```python
from build123d import *

# Parameters (mm, degrees)
SALIENTE_EXTRUIR1_DEPTH = 60
CORTAR_EXTRUIR1_REACH   = 50
CROQUIS2_R              = 2
CROQUIS2_R_2            = 12.5
SALIENTE_EXTRUIR2_DEPTH = 15
CROQUIS4_W              = 60
CROQUIS4_H              = 6
SALIENTE_EXTRUIR3_DEPTH = 1
CORTAR_EXTRUIR2_REACH   = 50
CROQUIS5_R              = 2.75
CROQUIS6_R              = 6
CORTAR_EXTRUIR3_DEPTH   = 8
REDONDEO1_R             = 5


with BuildPart() as part:
    # Croquis1 → Saliente-Extruir1 (new body)
    with BuildSketch(Plane.XY):
        Polygon((0, 0), (0, -30), (42, -30), (42, -90), (48, -90), (48, -21), (14, -21), (14, 0), align=None)
    extrude(amount=SALIENTE_EXTRUIR1_DEPTH)

    # Croquis2 → Cortar-Extruir1 (cut, up to next)
    with BuildSketch(Plane(origin=(48, 0, 0), x_dir=(0, 0, -1), z_dir=(1, 0, 0)), mode=Mode.PRIVATE) as cortar_extruir1_sk1:
        with Locations((-45.5, -44.5)):
            Circle(CROQUIS2_R)
    cortar_extruir1_tool1 = extrude(cortar_extruir1_sk1.sketch, amount=-CORTAR_EXTRUIR1_REACH, mode=Mode.PRIVATE) & part.part
    add(cortar_extruir1_tool1.solids().sort_by_distance((48, -44.5, 45.5))[0], mode=Mode.SUBTRACT)
    # Croquis2 → Cortar-Extruir1 (cut, up to next)
    with BuildSketch(Plane(origin=(48, 0, 0), x_dir=(0, 0, -1), z_dir=(1, 0, 0)), mode=Mode.PRIVATE) as cortar_extruir1_sk2:
        with Locations((-14.5, -44.5)):
            Circle(CROQUIS2_R)
    cortar_extruir1_tool2 = extrude(cortar_extruir1_sk2.sketch, amount=-CORTAR_EXTRUIR1_REACH, mode=Mode.PRIVATE) & part.part
    add(cortar_extruir1_tool2.solids().sort_by_distance((48, -44.5, 14.5))[0], mode=Mode.SUBTRACT)
    # Croquis2 → Cortar-Extruir1 (cut, up to next)
    with BuildSketch(Plane(origin=(48, 0, 0), x_dir=(0, 0, -1), z_dir=(1, 0, 0)), mode=Mode.PRIVATE) as cortar_extruir1_sk3:
        with Locations((-45.5, -75.5)):
            Circle(CROQUIS2_R)
    cortar_extruir1_tool3 = extrude(cortar_extruir1_sk3.sketch, amount=-CORTAR_EXTRUIR1_REACH, mode=Mode.PRIVATE) & part.part
    add(cortar_extruir1_tool3.solids().sort_by_distance((48, -75.5, 45.5))[0], mode=Mode.SUBTRACT)
    # Croquis2 → Cortar-Extruir1 (cut, up to next)
    with BuildSketch(Plane(origin=(48, 0, 0), x_dir=(0, 0, -1), z_dir=(1, 0, 0)), mode=Mode.PRIVATE) as cortar_extruir1_sk4:
        with Locations((-14.5, -75.5)):
            Circle(CROQUIS2_R)
    cortar_extruir1_tool4 = extrude(cortar_extruir1_sk4.sketch, amount=-CORTAR_EXTRUIR1_REACH, mode=Mode.PRIVATE) & part.part
    add(cortar_extruir1_tool4.solids().sort_by_distance((48, -75.5, 14.5))[0], mode=Mode.SUBTRACT)
    # Croquis2 → Cortar-Extruir1 (cut, up to next)
    with BuildSketch(Plane(origin=(48, 0, 0), x_dir=(0, 0, -1), z_dir=(1, 0, 0)), mode=Mode.PRIVATE) as cortar_extruir1_sk5:
        with Locations((-30, -60)):
            Circle(CROQUIS2_R_2)
    cortar_extruir1_tool5 = extrude(cortar_extruir1_sk5.sketch, amount=-CORTAR_EXTRUIR1_REACH, mode=Mode.PRIVATE) & part.part
    add(cortar_extruir1_tool5.solids().sort_by_distance((48, -60, 30))[0], mode=Mode.SUBTRACT)

    # Croquis3 → Saliente-Extruir2 (add)
    with BuildSketch(Plane.ZY.offset(-42)):
        Polygon((0, -30), (0, -90), (60, -90), (60, -30), (55, -30), (55, -85), (5, -85), (5, -30), align=None)
    extrude(amount=SALIENTE_EXTRUIR2_DEPTH)

    # Croquis4 → Saliente-Extruir3 (add)
    with BuildSketch(Plane(origin=(14, 0, 0), x_dir=(0, 0, -1), z_dir=(1, 0, 0))):
        with Locations((-30, -10)):
            Rectangle(CROQUIS4_W, CROQUIS4_H)
    extrude(amount=SALIENTE_EXTRUIR3_DEPTH)

    # Croquis5 → Cortar-Extruir2 (cut, up to next)
    with BuildSketch(Plane.ZY, mode=Mode.PRIVATE) as cortar_extruir2_sk1:
        with Locations((15, -10)):
            Circle(CROQUIS5_R)
    cortar_extruir2_tool1 = extrude(cortar_extruir2_sk1.sketch, amount=-CORTAR_EXTRUIR2_REACH, mode=Mode.PRIVATE) & part.part
    add(cortar_extruir2_tool1.solids().sort_by_distance((0, -10, 15))[0], mode=Mode.SUBTRACT)
    # Croquis5 → Cortar-Extruir2 (cut, up to next)
    with BuildSketch(Plane.ZY, mode=Mode.PRIVATE) as cortar_extruir2_sk2:
        with Locations((45, -10)):
            Circle(CROQUIS5_R)
    cortar_extruir2_tool2 = extrude(cortar_extruir2_sk2.sketch, amount=-CORTAR_EXTRUIR2_REACH, mode=Mode.PRIVATE) & part.part
    add(cortar_extruir2_tool2.solids().sort_by_distance((0, -10, 45))[0], mode=Mode.SUBTRACT)

    # Croquis6 → Cortar-Extruir3 (cut)
    with BuildSketch(Plane.ZY):
        with Locations((15, -10)):
            Circle(CROQUIS6_R)
        with Locations((45, -10)):
            Circle(CROQUIS6_R)
    extrude(amount=-CORTAR_EXTRUIR3_DEPTH, mode=Mode.SUBTRACT)

    # Redondeo1
    redondeo1_edges = [part.edges().sort_by_distance(p)[0] for p in [
        (13.5, -30, 60),
        (13.5, -30, 0),
    ]]
    fillet(redondeo1_edges, radius=REDONDEO1_R)


solid = part.part
```
Could you check a few things on this model? Use its own coordinates, in mm. A direction names the side the tool comes from. Round coordinates to 2 decimals unless told otherwise and drop trailing zeros. Order: outer loops, then holes, each group sorted by start corner. A loop starts at its lowest first (then second) coordinate and runs counter-clockwise, first axis right, second up. Notation, with made-up numbers: (87, 68.25) -> (143, 68.25) arc R22 ccw to (143, 104.25) -> close; hole circle Ø1 at (-7, -27). An arc over 180 degrees is marked (long way). One line per question, with ' | ' between items.
Q1. If we section it at D-D on x = 6: Write out the boundary of the cut face in (y, z), plus the area to 3 significant figures.
Computed values:
outline: (-30, 5) arc R5 ccw to (-25, 0) -> (0, 0) -> (0, 60) -> (-25, 60) arc R5 ccw to (-30, 55) -> close; hole circle Ø12 at (-10, 15); hole circle Ø12 at (-10, 45) | area: 1,560 mm²
Q2. If we section it at B-B on x = 29: Write out the boundary of the cut face in (y, z), plus the area to 3 significant figures.
Computed values:
outline: (-90, 0) -> (-21, 0) -> (-21, 60) -> (-90, 60) -> close; hole (-85, 5) -> (-30, 5) -> (-30, 55) -> (-85, 55) -> close | area: 1,390 mm²
Q3. If we section it at A-A on y = -60: Write out the boundary of the cut face in (x, z), plus the area to 3 significant figures.
Computed values:
outline: (27, 0) -> (48, 0) -> (48, 17.5) -> (42, 17.5) -> (42, 5) -> (27, 5) -> close; (27, 55) -> (42, 55) -> (42, 42.5) -> (48, 42.5) -> (48, 60) -> (27, 60) -> close | area: 360 mm²
Q4. If I drill on line 1 (Y direction, x = 13, z = 45); line 2 (Y direction, x = 44, z = 30); line 3 (Y direction, x = 46.4, z = 14.5), over which ranges is the centre line in solid material (lowest first)? Write a range as from..to.
Computed values:
line 1: -30..-12.75, -7.25..0 | line 2: -90..-72.5, -47.5..-21 | line 3: -90..-77.5, -73.5..-46.5, -42.5..-21
Q5. Which directions (+Z, -Z, +X, -X, +Y, -Y) give clear straight access to the entire face, cutting with the end or side of a thin tool? Please do faces 5 (the face through (14, -4, 30)), 6 (the face through (45.042, -46.452, 14.934)), 7 (the face through (14, -17, 30)), 8 (the face through (35, -57, 55)), 9 (the face through (14, -29, 58)).
Computed values:
face 5: +Z, -Z, +X, +Y | face 6: +X, -X | face 7: +Z, -Z, +X | face 8: -X | face 9: +Z, -X, -Y
Q6. We'd pull the mould along Y, two halves only. Please class faces 1 (the face through (11.451, -9.879, 42.253)), 2 (the face through (14, -28, 1)), 3 (the face through (27, -86, 30)), 4 (the face through (45.042, -73.517, 14.76)): released by +Y, released by -Y, zero draft, split by the parting line, or undercut.
Computed values:
face 1: undercut | face 2: released by -Y | face 3: zero draft | face 4: undercut
Q7. If we section it at C-C on z = 45.5: Give the number of separate pieces and of enclosed holes in the cut face, plus the area to 3 significant figures.
Computed values:
separate pieces: 4 | enclosed holes: 0 | area: 985 mm²
Q8. I'm going to push flat-ended pins straight in: pin 1 (10 mm diameter, centred on x = 24, z = 16, fed in from +Y); pin 2 (3.5 mm diameter, centred on y = -12.5, z = 16.5, fed in from -X); pin 3 (1.5 mm diameter, centred on y = -53, z = 39, fed in from +X); pin 4 (5 mm diameter, centred on y = -75.5, z = 38.5, fed in from -X). Where does each tip first touch, or does it pass through?
Computed values:
pin 1: y = -21 | pin 2: x = 8 | pin 3: through | pin 4: x = 42
